Geometry check sheet. Reference: drawing and pictorial views, mm from the part's lowest x, y, z. Give positions to 0.01 mm unless a question says otherwise; leave off trailing zeros. Write each loop counter-clockwise with the first axis right and the second up, starting at its lowest first coordinate (ties: lowest second). Pieces come first, ordered by that corner, then holes. Notation, with made-up numbers: M 33,53 L 49,53 A27 cw 49,87 Z; hole C -20,62 d9. An arc over 180 degrees is marked long. One line per item, written item: value. Start each with the question number.
1. Cross-section at C-C on y = 1.6. Record the cut outline in (x, z) (1 decimal), then the cut area to 3 significant figures.
2. Cross-section at A-A on x = 5. Record the cut outline in (y, z), then the cut area to 3 significant figures.
3. Cross-section at D-D on x = 29.5. Record the cut outline in (y, z).
4. Scan lines: line 1 (X direction, y = 1.95, z = 5) (1 decimal); line 2 (X direction, y = 1.45, z = 27.5) (1 decimal); line 3 (X direction, y = 2.5, z = 5.5) (1 decimal). Record each from-to range of solid material in increasing order.
5. Gauge pin test, flat end, axial feed: pin 1 (1 mm diameter, centred on x = 22.5, y = 1.5, fed in from -Z). Record the tip position at first contact, or that the pin passes through.
6. Cross-section at B-B on z = 24. Record the cut outline in (x, y) (1 decimal), then the cut area to 3 significant figures.
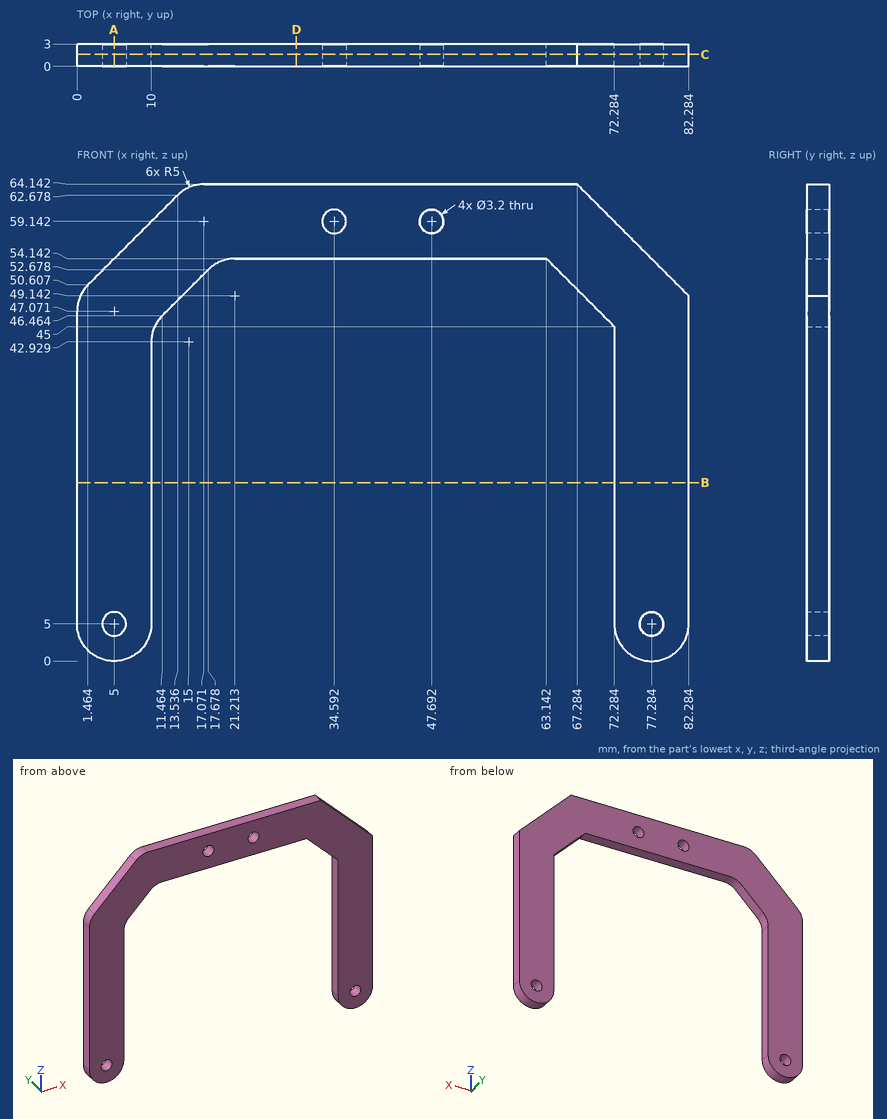
Report:
1. outline: M 0,5 A5 ccw 10,5 L 10,42.9 A5 cw 11.5,46.5 L 17.7,52.7 A5 cw 21.2,54.1 L 63.1,54.1 L 72.3,45 L 72.3,5 A5 ccw 82.3,5 L 82.3,49.1 L 67.3,64.1 L 17.1,64.1 A5 ccw 13.5,62.7 L 1.5,50.6 A5 ccw 0,47.1 Z; hole C 5,5 d3.2; hole C 34.6,59.1 d3.2; hole C 47.7,59.1 d3.2; hole C 77.3,5 d3.2
1. area: 1,710 mm^2
2. outline: M 0,0 L 3,0 L 3,3.4 L 0,3.4 Z; M 0,6.6 L 3,6.6 L 3,54.14 L 0,54.14 Z
2. area: 153 mm^2
3. outline: M 0,54.14 L 3,54.14 L 3,64.14 L 0,64.14 Z
4. line 1: x = 0 to 3.4, 6.6 to 10, 72.3 to 75.7, 78.9 to 82.3
4. line 2: x = 0 to 10, 72.3 to 82.3
4. line 3: x = 0 to 3.5, 6.5 to 10, 72.3 to 75.8, 78.8 to 82.3
5. pin 1: stops at z = 54.14
6. outline: M 0,0 L 10,0 L 10,3 L 0,3 Z; M 72.3,0 L 82.3,0 L 82.3,3 L 72.3,3 Z
6. area: 60.0 mm^2
